Here's the drawing with two shaded views (mm, measured from the low corner). I have some questions. A direction names the side the tool comes from. Give positions to 0.01 mm unless a question says otherwise; leave off trailing zeros. Write each loop counter-clockwise with the first axis right and the second up, starting at its lowest first coordinate (ties: lowest second). Pieces come first, ordered by that corner, then holes.
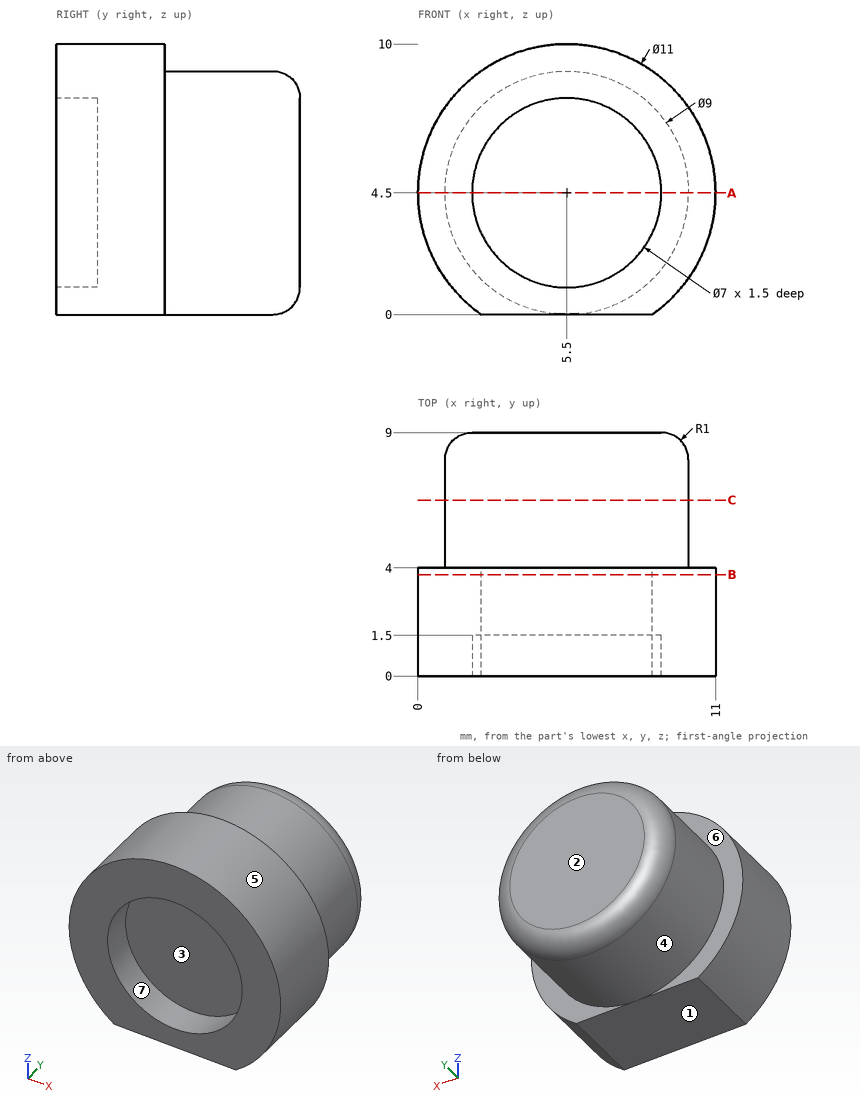
1) Suppose I cut it at A-A on z = 4.5. Write out the boundary of the cut face in (x, y), plus the area to 3 significant figures.
Values follow:
outline: (0, 0) - (2, 0) - (2, 1.5) - (9, 1.5) - (9, 0) - (11, 0) - (11, 4) - (10, 4) - (10, 8) arc R1 ccw to (9, 9) - (2, 9) arc R1 ccw to (1, 8) - (1, 4) - (0, 4) - close
area: 78.1 mm2
2) Suppose I cut it at C-C on y = 6.5. Write out the boundary of the cut face in (x, z).
Values follow:
outline: circle Ø9 at (5.5, 4.5)
3) For pin 1 Ø1.5 at (y, z) = (5, 5) entering from -X; pin 2 Ø2 at (y, z) = (1.5, 3.5) entering from +X; pin 3 Ø5.5 at (x, z) = (5.5, 4.5) entering from -Y, each with a flat end and sliding along its axis, tell me the tip position at first contact or that it passes through.
Values follow:
pin 1: stops at x = 1
pin 2: stops at x = 11
pin 3: stops at y = 1.5
4) For the marked faces 5, 6 and 7, which set-ups out of +Z, -Z, +X, -X, +Y, -Y let a thin tool reach every point of the face, with its end or its side?
Values follow:
face 5: +Y, -Y
face 6: +Y
face 7: -Y
5) If we mould it in two halves opening along Z, with no side actions, what happens to the marked faces 1, 2, 3 and 4? For each: +Z half, -Z half, draft (parallel to the pull), parting line (faces both ways), or undercut.
Values follow:
face 1: -Z half
face 2: draft
face 3: undercut
face 4: parting line
6) Please list where these lines run through material, in increasing order: L1, parallel to Z at x = 5.5, y = 0.55; L2, parallel to Y at x = 5.25, z = 1.25; L3, parallel to X at y = 1, z = 4.
Values follow:
L1: z = 0 to 1, 8 to 10
L2: y = 1.5 to 9
L3: x = 0.02 to 2.04, 8.96 to 10.98
7) Suppose I cut it at B-B on y = 3.75. Write out the boundary of the cut face in (x, z), plus the area to 3 significant figures.
Values follow:
outline: (2.34, 0) - (8.66, 0) arc R5.5 ccw (long way) to start
area: 90.7 mm2
